```python
from build123d import *

# Parameters (mm, degrees)
SKETCH1_R           = 5
SKETCH1_R_2         = 2
BOSS_EXTRUDE1_DEPTH = 2
SKETCH2_R           = 2
SKETCH2_R_2         = 5
BOSS_EXTRUDE2_DEPTH = 2
SKETCH3_R           = 3
SKETCH3_R_2         = 2.5
BOSS_EXTRUDE3_DEPTH = 46
BOSS_EXTRUDE5_DEPTH = 46
SKETCH7_R           = 5
SKETCH7_R_2         = 2.5
BOSS_EXTRUDE6_DEPTH = 5


with BuildPart() as part:
    # Sketch1 → Boss-Extrude1 (new body)
    with BuildSketch(Plane.XY):
        with BuildLine():
            Line((-15, 0), (15, 0))
            Line((15, 0), (10.788133888, 21.148526754))
            ThreePointArc((10.788133888, 21.148526754), (0, 30), (-10.788133888, 21.148526754))
            Line((-10.788133888, 21.148526754), (-15, 0))
        make_face()
        with Locations((0, 15)):
            Circle(SKETCH1_R, mode=Mode.SUBTRACT)
        with Locations((5, 8)):
            Circle(SKETCH1_R_2, mode=Mode.SUBTRACT)
        with Locations((-5, 8)):
            Circle(SKETCH1_R_2, mode=Mode.SUBTRACT)
        with Locations((0, 25)):
            Circle(SKETCH1_R_2, mode=Mode.SUBTRACT)
    extrude(amount=BOSS_EXTRUDE1_DEPTH)



with BuildPart() as body_2:
    # Sketch2 → Boss-Extrude2 (new body)
    with BuildSketch(Plane(origin=(0, 0, 50), x_dir=(-1, 0, 0), z_dir=(0, 0, -1))):
        with BuildLine():
            Line((-10.788133888, 21.148526754), (-15, 0))
            Line((-15, 0), (15, 0))
            Line((15, 0), (10.788133888, 21.148526754))
            ThreePointArc((10.788133888, 21.148526754), (0, 30), (-10.788133888, 21.148526754))
        make_face()
        with Locations(Location((-5, 8, 0), (0, 0, 180))):
            Circle(SKETCH2_R, mode=Mode.SUBTRACT)
        with Locations(Location((5, 8, 0), (0, 0, 180))):
            Circle(SKETCH2_R, mode=Mode.SUBTRACT)
        with Locations(Location((0, 25, 0), (0, 0, 180))):
            Circle(SKETCH2_R, mode=Mode.SUBTRACT)
        with Locations(Location((0, 15, 0), (0, 0, 180))):
            Circle(SKETCH2_R_2, mode=Mode.SUBTRACT)
    extrude(amount=BOSS_EXTRUDE2_DEPTH)


with BuildPart() as part_1:
    add(part.part)

    add(body_2.part)  # Boss-Extrude3 merges body 2
    # Sketch3 → Boss-Extrude3 (add)
    # profile 1 of 3: a face of its own
    with BuildSketch(Plane.XY.offset(2)):
        with Locations(Location((5, 8, 0), (0, 0, 180))):
            Circle(SKETCH3_R)
        with Locations(Location((5, 8, 0), (0, 0, 180))):
            Circle(SKETCH3_R_2, mode=Mode.SUBTRACT)
    # profile 2 of 3: a face of its own
    with BuildSketch(Plane.XY.offset(2)):
        with Locations(Location((0, 25, 0), (0, 0, 180))):
            Circle(SKETCH3_R)
        with Locations(Location((0, 25, 0), (0, 0, 180))):
            Circle(SKETCH3_R_2, mode=Mode.SUBTRACT)
    # profile 3 of 3: a face of its own
    with BuildSketch(Plane.XY.offset(2)):
        with Locations(Location((-5, 8, 0), (0, 0, 180))):
            Circle(SKETCH3_R)
        with Locations(Location((-5, 8, 0), (0, 0, 180))):
            Circle(SKETCH3_R_2, mode=Mode.SUBTRACT)
    extrude(amount=BOSS_EXTRUDE3_DEPTH)

    # Sketch4 → Boss-Extrude5 (add)
    with BuildSketch(Plane.XY.offset(2)):
        Polygon((-10.788133888, 21.148526754), (-14.203374086, 4), (-10.124818846, 4), (-6.709578648, 21.148526754), align=None)
        Polygon((10.124818846, 4), (14.203374086, 4), (10.788133888, 21.148526754), (6.709578648, 21.148526754), align=None)
        Polygon((-14.203374086, 4), (-15, 0), (15, 0), (14.203374086, 4), (10.124818846, 4), (-10.124818846, 4), align=None)
    extrude(amount=BOSS_EXTRUDE5_DEPTH)

    # Sketch7 → Boss-Extrude6 (add)
    # profile 1 of 4: a face of its own
    with BuildSketch(Plane.XZ):
        with Locations(Location((7.5, 37.5, 0), (0, 0, 90))):
            Circle(SKETCH7_R)
        with Locations(Location((7.5, 37.5, 0), (0, 0, 270))):
            Circle(SKETCH7_R_2, mode=Mode.SUBTRACT)
    # profile 2 of 4: a face of its own
    with BuildSketch(Plane.XZ):
        with Locations(Location((7.5, 12.5, 0), (0, 0, 90))):
            Circle(SKETCH7_R)
        with Locations(Location((7.5, 12.5, 0), (0, 0, 90))):
            Circle(SKETCH7_R_2, mode=Mode.SUBTRACT)
    # profile 3 of 4: a face of its own
    with BuildSketch(Plane.XZ):
        with Locations(Location((-7.5, 12.5, 0), (0, 0, 90))):
            Circle(SKETCH7_R)
        with Locations(Location((-7.5, 12.5, 0), (0, 0, 270))):
            Circle(SKETCH7_R_2, mode=Mode.SUBTRACT)
    # profile 4 of 4: a face of its own
    with BuildSketch(Plane.XZ):
        with Locations(Location((-7.5, 37.5, 0), (0, 0, 90))):
            Circle(SKETCH7_R)
        with Locations(Location((-7.5, 37.5, 0), (0, 0, 90))):
            Circle(SKETCH7_R_2, mode=Mode.SUBTRACT)
    extrude(amount=BOSS_EXTRUDE6_DEPTH)


solid = part_1.part
```
Read the model definition and answer for the solid it produces. Units are mm, in the model's axes. A direction names the side the tool comes from. Coordinates: 2 decimals unless noted, no trailing zeros. Write each loop counter-clockwise with the first axis right and the second up, starting at its lowest first coordinate (ties: lowest second). Pieces come first, ordered by that corner, then holes. Notation, with made-up numbers: (7.5, -17) -> (65.5, -17) arc R27 ccw to (65.5, 14) -> close; hole circle Ø7 at (83.5, 88). An arc over 180 degrees is marked (long way). Answer as a JSON object with one key per item and string values.
Q1. The part is cut by section B-B on z = 22. Give the vertices of the cut face in (x, y).
The answers:
{"outline": "(-15, 0) -> (15, 0) -> (10.79, 21.15) -> (6.71, 21.15) -> (10.12, 4) -> (-10.12, 4) -> (-6.71, 21.15) -> (-10.79, 21.15) -> close; circle Ø6 at (-5, 8); circle Ø6 at (0, 25); circle Ø6 at (5, 8); hole circle Ø5 at (-5, 8); hole circle Ø5 at (0, 25); hole circle Ø5 at (5, 8)"}
Q2. The part is cut by section A-A on y = -1. Give the vertices of the cut face in (x, z), then the cut area to 3 significant figures.
The answers:
{"outline": "circle Ø10 at (-7.5, 12.5); circle Ø10 at (-7.5, 37.5); circle Ø10 at (7.5, 12.5); circle Ø10 at (7.5, 37.5); hole circle Ø5 at (-7.5, 12.5); hole circle Ø5 at (-7.5, 37.5); hole circle Ø5 at (7.5, 12.5); hole circle Ø5 at (7.5, 37.5)", "area": "236 mm2"}
Q3. Determine the mould class of faces 1 (the flat face through (7, 0, 12)), 2 (the cylindrical face through (0, 30, 1)) for opening direction Z: pulls with the +Z half, pulls with the -Z half, needs draft (parallel to the pull), parting line crosses it, or undercut.
The answers:
{"face 1": "undercut", "face 2": "needs draft"}
Q4. Flat-ended cylindrical pins translate along their axes: pin 1 Ø4 at (y, z) = (2.5, 36.5) entering from +X; pin 2 Ø2.5 at (x, y) = (-5, 8) entering from +Z; pin 3 Ø1.5 at (x, z) = (-6, 36.5) entering from +Y; pin 4 Ø9 at (x, z) = (-3.5, 28.5) entering from -Y. Find the tip coordinate at first contact, or state that the pin passes through.
The answers:
{"pin 1": "stops at x = 14.9", "pin 2": "passes through", "pin 3": "stops at y = 21.15", "pin 4": "stops at y = 0"}
Q5. Consider line 1 (Y direction, x = 0, z = 49.3); line 2 (X direction, y = -0.95, z = 37.5); line 3 (Y direction, x = -6, z = 6.5). Determine where each line is inside the solid, lowest interval first. Write a range as [from, to].
The answers:
{"line 1": "y = [0, 10], [20, 23], [27, 30]", "line 2": "x = [-12.5, -10], [-5, -2.5], [2.5, 5], [10, 12.5]", "line 3": "y = [0, 4], [5.17, 5.71], [10.29, 10.83]"}
Q6. The part is cut by section C-C on x = 0. Give the number of separate pieces and of enclosed holes in the cut face, then the cut area to 3 significant figures.
The answers:
{"separate pieces": "3", "enclosed holes": "0", "area": "294 mm2"}
Q7. The part is cut by section D-D on y = 26. Give the vertices of the cut face in (x, z), then the cut area to 3 significant figures.
The answers:
{"outline": "(-8.49, 0) -> (-1.73, 0) -> (-1.73, 2) -> (-2.29, 2) -> (-2.29, 48) -> (-1.73, 48) -> (-1.73, 50) -> (-8.49, 50) -> (-8.49, 48) -> (-2.83, 48) -> (-2.83, 2) -> (-8.49, 2) -> close; (1.73, 0) -> (8.49, 0) -> (8.49, 2) -> (2.83, 2) -> (2.83, 48) -> (8.49, 48) -> (8.49, 50) -> (1.73, 50) -> (1.73, 48) -> (2.29, 48) -> (2.29, 2) -> (1.73, 2) -> close", "area": "103 mm2"}
Q8. A tool of negligible diameter and unlimited length cuts with its end or side. For faces 3 (the cylindrical face through (9, -2.5, 10.5)), 4 (the cylindrical face through (-6.474, 6.648, 49.014)), 5 (the cylindrical face through (0.33, 22.52, 24.68)), from which of +Z, -Z, +X, -X, +Y, -Y can it reach the whole face along a straight path? Write none if from no direction.
The answers:
{"face 3": "-Y", "face 4": "+Z, -Z", "face 5": "none"}
